Autodesk Inventor part; units mm, degrees
ref_plane "YZ Plane" through (0, 0, 0) normal (1, 0, 0) x (0, 1, 0)
ref_plane "XZ Plane" through (0, 0, 0) normal (0, 1, 0) x (-1, 0, 0)
ref_plane "XY Plane" through (0, 0, 0) normal (0, 0, 1) x (1, 0, 0)
sketch "Sketch1" plane through (0, 0, 0) normal (0, 0, 1) x (1, 0, 0)
  line L0 (-35.5537, 46.3091) -> (69.62, 46.3091) construction
  line L1 (69.62, 46.3091) -> (69.62, -40.915) construction
  line L2 (69.62, -40.915) -> (-35.5537, -40.915) construction
  line L3 (-35.5537, -40.915) -> (-35.5537, 46.3091) construction
  line L4 (-11.5, -3.1187) -> (11.5, -3.1187)
  point P0 (0, 0)
  point P1 (0, 0)
  dimension "d19" = 23
sketch "Sketch5" plane through (0, 0, 0) normal (0, 1, 0) x (-1, 0, 0)
  line L0 (-51.6883, 69.5392) -> (52.6581, 69.5392) construction
  line L1 (52.6581, 69.5392) -> (52.6581, -16.9988) construction
  line L2 (52.6581, -16.9988) -> (-51.6883, -16.9988) construction
  line L3 (-51.6883, -16.9988) -> (-51.6883, 69.5392) construction
  line L4 (16, 8.395) -> (-16, 8.395)
  circle A0 centre (-5.616, 0) radius 2.5
  circle A1 centre (-5.616, 0) radius 4.5
  circle A2 centre (-13.9015, 3.5026) radius 1.25
  line L5 (-5.616, 0) -> (-20.9236, 0)
  circle A3 centre (-13.9015, -3.5026) radius 1.25
  line L6 (0, 0) -> (0, -9.2667)
  circle A4 centre (13.9015, 3.5026) radius 1.25
  circle A5 centre (13.9015, -3.5026) radius 1.25
  line L7 (13.9015, -3.5026) -> (13.9015, 3.5026)
  arc A6 (13.9015, 1.0292) -> (13.9015, -0.9708) centre (13.9015, 0.0292) ccw
  line L8 (13.9015, -0.9708) -> (16.5074, -0.9708)
  line L9 (16.5074, 1.0292) -> (13.9015, 1.0292)
  line L10 (16.5074, -0.9708) -> (16.5074, 1.0292)
  point P0 (0, 8.395)
  dimension "d30" = 32
  dimension "d57" = 9
  dimension "d58" = 5
  dimension "d63" = 2.5
  dimension "d83" = 2
  dimension "d84" = 1
sketch "Sketch6" plane through (0, 0, 0) normal (0, 1, 0) x (-1, 0, 0)
  line L0 (11.515, 6.0048) -> (11.515, -5.9952)
  line L1 (11.515, 0.0048) -> (-11.485, 0.0048)
  line L2 (11.515, -5.9952) -> (11.515, 6.0048)
  line L3 (-11.485, 6.0048) -> (-11.485, -5.9952)
  line L4 (11.515, -5.9952) -> (-11.485, -5.9952)
  line L5 (-11.485, 6.0048) -> (11.515, 6.0048)
  point P0 (0, 0)
  point P1 (9.3248, 11.448)
  point P2 (-11.485, 0.0048)
  dimension "d42" = 12
  dimension "d43" = 23
  dimension "d44" = 12
extrude "Extrusion1" add sketch "Sketch6" along normal blind 26.3
extrude "Extrusion2" add sketch "Sketch5" along normal blind 1 from surface at 26.3 contours A0 | A1
sketch "Sketch7" plane through (-11.515, 0, -5.9952) normal (-1, 0, 0) x (0, 0, 1)
  line L0 (5.9952, 0) -> (5.9952, 19.8)
  line L1 (5.9952, 19.8) -> (5.9952, 20.8)
  line L2 (0, 0) -> (0, 26.3)
  line L3 (0, 19.8) -> (12, 19.8)
  line L4 (12, 0) -> (12, 26.3)
  line L5 (12, 20.8) -> (0, 20.8)
  line L6 (0, 20.8) -> (0, 19.8)
  dimension "d49" = 19.8
  dimension "d50" = 1
extrude "Extrusion3" add sketch "Sketch7" along normal blind 4.5
sketch "Sketch8" plane through (11.485, 0, 6.0048) normal (1, 0, 0) x (0, 0, -1)
  line L0 (6.0048, 0) -> (6.0048, 19.8)
  line L1 (6.0048, 19.8) -> (6.0048, 20.8)
  line L2 (0, 0) -> (0, 26.3)
  line L3 (0, 19.7999) -> (12, 19.7999)
  line L4 (12, 20.8) -> (12, 19.8)
  line L5 (12, 19.7999) -> (12, 20.8)
  line L6 (12, 20.8) -> (0, 20.8)
  line L7 (0, 20.8) -> (0, 19.7999)
  dimension "d53" = 19.8
  dimension "d54" = 1
extrude "Extrusion4" add sketch "Sketch8" along normal blind 4.5
extrude "Extrusion5" add sketch "Sketch5" along normal blind 3.7 from surface at 27.3 contours A0
fillet "Fillet1" radius 1 12 edges at (11.485, 9.8999, 6.0048) (11.485, 9.8999, -5.9952) (-11.515, 9.9, -5.9952) (-11.515, 23.55, -5.9952) (-11.515, 23.55, 6.0048) (-11.515, 9.9, 6.0048) (-16.015, 20.3, 6.0048) (-16.015, 20.3, -5.9952) (11.485, 23.55, -5.9952) (15.985, 20.2999, -5.9952) (15.985, 20.2999, 6.0048) (11.485, 23.55, 6.0048)
extrude "Extrusion6" cut sketch "Sketch5" along normal up to surface (20.8 mm away) contours A2
extrude "Extrusion7" cut sketch "Sketch5" along normal up to surface (20.8 mm away) contours A3
extrude "Extrusion8" cut sketch "Sketch5" along normal up to surface (20.8 mm away) contours A4
extrude "Extrusion9" cut sketch "Sketch5" along normal up to surface (20.8 mm away) contours A5
sketch "Sketch9" plane through (11.485, 0, 5.0048) normal (1, 0, 0) x (0, 0, -1)
  line L0 (10, 26.3) -> (10, 20.8)
  line L1 (11, 0) -> (10, 0)
  line L2 (10, 26.3) -> (10, 0)
  line L3 (10, 19.7999) -> (10, 0)
  line L4 (0, 0) -> (0, 19.7999)
  line L5 (5.0048, 0) -> (5.0048, 5)
  line L6 (5.0048, 5) -> (5.0048, 8.5)
  line L7 (5.0048, 5) -> (8.0048, 5)
  line L8 (5.0048, 5) -> (2.0048, 5)
  line L9 (2.0048, 5) -> (2.0048, 8.5)
  line L10 (2.0048, 8.5) -> (8.0048, 8.5)
  line L11 (8.0048, 8.5) -> (8.0048, 5)
  dimension "d76" = 26.3
  dimension "d77" = 5
  dimension "d78" = 3.5
  dimension "d79" = 3
extrude "Extrusion10" add sketch "Sketch9" along normal blind 1
extrude "Extrusion11" cut sketch "Sketch5" along normal up to surface (20.8 mm away) contours L9 L10 L8 L7 | L7 A6
mirror "Spiegeln1" about plane through (0, 0, 0) normal (1, 0, 0) of "Extrusion11"
ref_plane "Arbeitsebene1" through (0, 0, 0) normal (1, 0, 0) x (0, 1, 0)
properties part number "servo_alzrc_ds452mg" material "Thermoplastic Resin"
Can you work these out from the model? Positions are in its coordinate system, mm. A direction names the side the tool comes from. Give positions to 0.01 mm unless a question says otherwise; leave off trailing zeros. Order: outer loops, then holes, each group sorted by start corner. A loop starts at its lowest first (then second) coordinate and runs counter-clockwise, first axis right, second up. Notation, with made-up numbers: M 84.25,2 L 97.25,2 A26 ccw 97.25,35 Z; hole C 30,80 d10. An arc over 180 degrees is marked long. Use one line per item in the form item = value. Start each with the question number.
Item 1: For faces 5 (the cylindrical face through (-11.23, 23.588, 5.704)), 6 (the cylindrical face through (-11.214, 10.039, -5.71)), 7 (the flat face through (3.7, 27.3, -1.9)), 8 (the flat face through (12, 7, 3)), which set-ups out of +Z, -Z, +X, -X, +Y, -Y let a thin tool reach every point of the face, with its end or its side?
Item 2: If we section it at D-D (z = 0): Write out the boundary of the cut face in (x, y) (3 decimals).
Item 3: Will these pins go through, and if not, where does the flat tip stop? pin 1 Ø1 at (y, z) = (6.5, 0.5) entering from +X (3 decimals); pin 2 Ø4.5 at (y, z) = (25, -1.5) entering from -X (3 decimals); pin 3 Ø4 at (x, z) = (-9.5, 0.5) entering from +Y.
Item 4: If we section it at A-A (y = 16.5): Write out the boundary of the cut face in (x, z) (3 decimals), then the cut area to 3 significant figures.
Item 5: If we section it at C-C (x = 13.5): Write out the boundary of the cut face in (y, z), then the cut area to 3 significant figures.
Item 6: If I drill on line 1 along X through (y, z) = (20, 2.5) (3 decimals); line 2 along Y through (x, z) = (-3, -0.75); line 3 along X through (y, z) = (22, 1) (3 decimals), over which ranges is the centre line in solid material (lowest first)?
Item 7: If we section it at B-B (x = -11): Write out the boundary of the cut face in (y, z).
Item 8: We'd pull the mould along Z, two halves only. Please class faces 1 (the cylindrical face through (11.184, 10.039, 5.72)), 2 (the flat face through (-15, 20, -0.971)), 3 (the flat face through (-15, 20, 1.029)), 4 (the flat face through (12, 7, -3)): +Z half, -Z half, draft (parallel to the pull), parting line (faces both ways), or undercut.
Outcome:
q1.face_5 = +Z, -X, +Y
q1.face_6 = -Z, -X, -Y
q1.face_7 = +Y
q1.face_8 = +Z, +X, -Y
q2.outline = M -12.902,19.8 L -11.515,19.8 L -11.515,0 L 11.485,0 L 11.485,5 L 12.485,5 L 12.485,8.5 L 11.485,8.5 L 11.485,19.8 L 12.902,19.8 L 12.902,20.8 L 11.485,20.8 L 11.485,26.3 L 10.116,26.3 L 10.116,27.3 L 8.116,27.3 L 8.116,31 L 3.116,31 L 3.116,27.3 L 1.116,27.3 L 1.116,26.3 L -11.515,26.3 L -11.515,20.8 L -12.902,20.8 Z
q3.pin_1 = 12.485
q3.pin_2 = -11.515
q3.pin_3 = 26.3
q4.outline = M -11.515,-4.995 A1 ccw -10.515,-5.995 L 10.485,-5.995 A1 ccw 11.485,-4.995 L 11.485,5.005 A1 ccw 10.485,6.005 L -10.515,6.005 A1 ccw -11.515,5.005 Z
q4.area = 275 mm2
q5.outline = M 19.8,-6 L 20.8,-6 L 20.8,-4.69 L 19.8,-4.69 Z; M 19.8,-2.32 L 20.8,-2.32 L 20.8,-0.89 L 19.8,-0.89 Z; M 19.8,0.95 L 20.8,0.95 L 20.8,2.32 L 19.8,2.32 Z; M 19.8,4.69 L 20.8,4.69 L 20.8,6 L 19.8,6 Z
q5.area = 5.43 mm2
q6.line_1 = -16.015 to -14.648, -13.155 to 13.155, 14.648 to 15.985
q6.line_2 = 0 to 26.3
q6.line_3 = -11.515 to 11.485
q7.outline = M 0,-5.87 L 19.8,-5.87 L 19.8,-6 L 20.8,-6 L 20.8,-5.87 L 26.3,-5.87 L 26.3,5.88 L 20.8,5.88 L 20.8,6 L 19.8,6 L 19.8,5.88 L 0,5.88 Z
q8.face_1 = +Z half
q8.face_2 = undercut
q8.face_3 = undercut
q8.face_4 = -Z half
